Geometry check sheet. Reference: the model listing, model coordinates, mm. A direction names the side the tool comes from. Give positions to 0.01 mm unless a question says otherwise; leave off trailing zeros. Loops run counter-clockwise (first coordinate to the right, second up) from the corner with the lowest first, then second, coordinate; pieces in that order, holes last.
1. Material ranges on L1, parallel to Y at x = -29.5, z = 1.6; L2, parallel to Y at x = 147, z = 2.35; L3, parallel to Y at x = 62.5, z = 2.85, recorded low to high.
2. Tool access check on faces 1 (the flat face through (-86, 15, 2)), 2 (the flat face through (90, 25, 3)), 3 (the flat face through (120, 35, 2)). Record the directions out of +Z, -Z, +X, -X, +Y, -Y that give a thin tool (end or side, any length) a straight path to the whole face; none if there is none.
3. Go/stop test with flat-tipped pins: pin 1 Ø8 at (x, y) = (111.5, 9) entering from -Z; pin 2 Ø2 at (y, z) = (32.5, 1) entering from -X. Record where each tip stops, or that it passes through.
4. Release check for a two-part mould opening along Y. For faces 4 (the flat face through (-2, -15, 2)), 5 (the flat face through (24, 72, 3)), 6 (the cylindrical face through (34.28, 28.314, 2.465)) record: +Y half, -Y half, draft (parallel to the pull), parting line (faces both ways), or undercut.
5. Cross-section at B-B, the plane x = -75. Record the cut outline in (y, z), plus the area to 3 significant figures.
6. Cross-section at A-A, the plane z = 1.7. State how many separate pieces and enclosed holes the cut face has, plus the area to 4 significant figures.
from build123d import *

# Parameters (mm, degrees)
SKETCH_1_W                 = 300
SKETCH_1_H                 = 30
EXTRUDE_1_DEPTH            = 5
HOLE_WIZARD_M3_1_D         = 3.2
M3X0_5_1_D                 = 2.5
HOLE_WIZARD_M4_2_D         = 4.3
M4X0_7_2_D                 = 3.3
PATTERN_LINEAR_1_COUNT     = 6
PATTERN_LINEAR_1_PITCH     = 25
PATTERN_LINEAR_1_COL_COUNT = 7
PATTERN_LINEAR_1_COL_PITCH = 25
EXTRUDE_3_DEPTH            = 5
SKETCH_13_R                = 3.6
CUT_EXTRUDE_2_DEPTH        = 160.843673631
M4X0_7_3_D                 = 3.3
HOLE_WIZARD_M4_1_D         = 4.3
SKETCH_26_W                = 22
SKETCH_26_H                = 5
EXTRUDE_4_DEPTH            = 30
M3X0_5_2_D                 = 2.5
HOLE_WIZARD_M3_2_D         = 3.2
FILLET_2_R                 = 5
SKETCH_36_R                = 8
CUT_EXTRUDE_3_DEPTH        = 173.481883107
PATTERN_LINEAR_3_COUNT     = 3
PATTERN_LINEAR_3_PITCH     = 15
SKETCH_40_W                = 60
SKETCH_40_H                = 5
EXTRUDE_6_DEPTH            = 20
M3X0_5_3_D                 = 2.5
FILLET_3_R                 = 10


with BuildPart() as part:
    # 草圖1 → 填料-伸長1 (new body)
    with BuildSketch(Plane.XY):
        Rectangle(SKETCH_1_W, SKETCH_1_H)
    extrude(amount=EXTRUDE_1_DEPTH)

    # M3 餘隙孔1 (through all)
    with Locations(Plane.XY.offset(5)):
        with Locations((0, -10), (0, 10), (-20, -10), (-20, 10)):
            Hole(HOLE_WIZARD_M3_1_D / 2)

    # M3x0.5 螺紋孔1 (through all)
    with Locations(Plane.XY.offset(5)):
        with Locations((-12.5, 0)):
            m3x0_5_1 = Hole(M3X0_5_1_D / 2)

    # M4 餘隙孔2 (through all)
    with Locations(Plane.XY.offset(5)):
        with Locations((52, -10), (52, 10)):
            hole_wizard_m4_2 = Hole(HOLE_WIZARD_M4_2_D / 2)

    # M4x0.7 螺紋孔2 (through all)
    with Locations(Plane.XY.offset(5)):
        with Locations((-126, 10), (-126, -10)):
            m4x0_7_2 = Hole(M4X0_7_2_D / 2)

    # 直線複製排列1: M3x0.5 螺紋孔1 ×6
    with Locations(*[(-i * PATTERN_LINEAR_1_PITCH, 0, 0) for i in range(1, PATTERN_LINEAR_1_COUNT)]):
        add(m3x0_5_1, mode=Mode.SUBTRACT)

    # 直線複製排列1 col: M3x0.5 螺紋孔1 ×7
    with Locations(*[(i * PATTERN_LINEAR_1_COL_PITCH, 0, 0) for i in range(1, PATTERN_LINEAR_1_COL_COUNT)]):
        add(m3x0_5_1, mode=Mode.SUBTRACT)

    # 鏡射1: M4x0.7 螺紋孔2 across plane
    add(m4x0_7_2.mirror(Plane(origin=(0, 0, 0), x_dir=(0, 0, 1), z_dir=(1, 0, 0))), mode=Mode.SUBTRACT)

    # 草圖16 → 填料-伸長3 (add, through all)
    with BuildSketch(Plane.XY):
        with BuildLine():
            Line((-20, 15), (46, 15))
            Line((46, 15), (46, 55))
            Line((46, 55), (0, 55))
            ThreePointArc((0, 55), (-14.142135624, 49.142135624), (-20, 35))
            Line((-20, 35), (-20, 15))
        make_face()
    extrude(amount=EXTRUDE_3_DEPTH)

    # 草圖13 → 除料-伸長2 (cut, through all)
    with BuildSketch(Plane.XY):
        with Locations(Location((33.5, 24.8, 0), (0, 0, 180))):
            Circle(SKETCH_13_R)
    extrude(amount=CUT_EXTRUDE_2_DEPTH, mode=Mode.SUBTRACT)

    # M4x0.7 螺紋孔3 (through all)
    with Locations(Plane.XY.offset(5)):
        with Locations((15, 22), (-15, 22)):
            Hole(M4X0_7_3_D / 2)

    # M4 餘隙孔1 (through all)
    with Locations(Plane.XY.offset(5)):
        with Locations((-29.5, -10), (-29.5, 10), (-53.5, -10), (-53.5, 10)):
            Hole(HOLE_WIZARD_M4_1_D / 2)

    # 草圖26 → 填料-伸長4 (add)
    with BuildSketch(Plane(origin=(0, 55, 0), x_dir=(1, 0, 0), z_dir=(0, 1, 0))):
        with Locations((35, -2.5)):
            Rectangle(SKETCH_26_W, SKETCH_26_H)
    extrude(amount=EXTRUDE_4_DEPTH)

    # M3x0.5 螺紋孔2 (through all)
    with Locations(Plane.XY.offset(5)):
        with Locations((35, 74), (35, 66)):
            Hole(M3X0_5_2_D / 2)

    # M3 餘隙孔2 (through all)
    with Locations(Plane.XY.offset(5)):
        with Locations((25, 24.8), (42, 24.8)):
            Hole(HOLE_WIZARD_M3_2_D / 2)

    # 圓角2
    fillet_2_edges = [part.edges().sort_by_distance(p)[0] for p in [
        (46, 85, 2.5),
        (24, 85, 2.5),
    ]]
    fillet(fillet_2_edges, radius=FILLET_2_R)

    # 草圖36 → 除料-伸長3 (cut, through all)
    with BuildSketch(Plane.XY.offset(5)):
        with Locations((31, 47)):
            Circle(SKETCH_36_R)
    extrude(amount=-CUT_EXTRUDE_3_DEPTH, mode=Mode.SUBTRACT)

    # 直線複製排列3: M4 餘隙孔2 ×3
    with Locations(*[(i * PATTERN_LINEAR_3_PITCH, 0, 0) for i in range(1, PATTERN_LINEAR_3_COUNT)]):
        add(hole_wizard_m4_2, mode=Mode.SUBTRACT)

    # 草圖40 → 填料-伸長6 (add)
    with BuildSketch(Plane(origin=(0, 15, 0), x_dir=(1, 0, 0), z_dir=(0, 1, 0))):
        with Locations((120, -2.5)):
            Rectangle(SKETCH_40_W, SKETCH_40_H)
    extrude(amount=EXTRUDE_6_DEPTH)

    # M3x0.5 螺紋孔3 (through all)
    with Locations(Plane(origin=(0, 0, 0), x_dir=(-1, 0, 0), z_dir=(0, 0, -1))):
        with Locations((-147, 32), (-93, 8), (-147, 8), (-93, 32)):
            Hole(M3X0_5_3_D / 2)

    # 圓角3
    fillet_3_edges = [part.edges().sort_by_distance(p)[0] for p in [
        (24, 55, 2.5),
    ]]
    fillet(fillet_3_edges, radius=FILLET_3_R)


solid = part.part
Result:
1. L1: y = -15 to -12.15, -7.85 to 7.85, 12.15 to 15
1. L2: y = -15 to 6.75, 9.25 to 30.75, 33.25 to 35
1. L3: y = -15 to -1.25, 1.25 to 15
2. face 1: +Z, -Z, -X, +Y
2. face 2: +Z, -Z, +Y
2. face 3: +Z, -Z, +X, +Y
3. pin 1: stops at z = 0
3. pin 2: stops at x = -20
4. face 4: -Y half
4. face 5: draft
4. face 6: undercut
5. outline: (-15, 0) - (15, 0) - (15, 5) - (-15, 5) - close
5. area: 150 mm2
6. separate pieces: 1
6. enclosed holes: 42
6. area: 12,850 mm2
